Autodesk Inventor part; units mm, degrees
ref_plane "YZ Plane" through (0, 0, 0) normal (1, 0, 0) x (0, 1, 0)
ref_plane "XZ Plane" through (0, 0, 0) normal (0, 1, 0) x (-1, 0, 0)
ref_plane "XY Plane" through (0, 0, 0) normal (0, 0, 1) x (1, 0, 0)
sketch "Sketch4" plane through (0, 0, 0) normal (0, 1, 0) x (-1, 0, 0)
  line L0 (0, 0) -> (59.7662, 0)
  line L1 (59.7662, 0) -> (59.7662, -146.1262)
  line L2 (59.7662, -146.1262) -> (0, -146.1262)
  line L3 (0, -146.1262) -> (0, 0)
  line L4 (59.7662, 0) -> (53.4924, 0)
  line L5 (53.4924, 0) -> (53.4924, -9.5758)
  line L6 (53.4924, -9.5758) -> (59.7662, -9.5758)
  line L7 (59.7662, -9.5758) -> (59.7662, 0)
  line L8 (53.4924, -9.5758) -> (45.8724, -9.5758)
  line L9 (45.8724, -9.5758) -> (45.8724, -24.8158)
  line L10 (45.8724, -24.8158) -> (53.4924, -24.8158)
  line L11 (53.4924, -24.8158) -> (53.4924, -9.5758)
  line L12 (45.8724, -24.8158) -> (45.8724, -37.5158)
  line L13 (45.8724, -37.5158) -> (53.4924, -37.5158)
  line L14 (53.4924, -37.5158) -> (53.4924, -52.7558)
  line L15 (53.4924, -52.7558) -> (45.8724, -52.7558)
  line L16 (45.8724, -52.7558) -> (45.8724, -37.5158)
  line L17 (45.8724, -52.7558) -> (45.8724, -65.4558)
  line L18 (45.8724, -65.4558) -> (53.4924, -65.4558)
  line L19 (53.4924, -65.4558) -> (53.4924, -80.6958)
  line L20 (53.4924, -80.6958) -> (45.8724, -80.6958)
  line L21 (45.8724, -80.6958) -> (45.8724, -65.4558)
  line L22 (45.8724, -80.6958) -> (45.8724, -93.3958)
  line L23 (45.8724, -93.3958) -> (53.4924, -93.3958)
  line L24 (53.4924, -93.3958) -> (53.4924, -108.6358)
  line L25 (53.4924, -108.6358) -> (45.8724, -108.6358)
  line L26 (45.8724, -108.6358) -> (45.8724, -93.3958)
  line L27 (45.8724, -108.6358) -> (45.8724, -121.3358)
  line L28 (45.8724, -121.3358) -> (53.4924, -121.3358)
  line L29 (53.4924, -121.3358) -> (53.4924, -136.5758)
  line L30 (53.4924, -136.5758) -> (45.8724, -136.5758)
  line L31 (45.8724, -136.5758) -> (45.8724, -121.3358)
  line L32 (0, 0) -> (7.1628, 0)
  line L33 (7.1628, 0) -> (7.1628, -9.5758)
  line L34 (7.1628, -9.5758) -> (0, -9.5758)
  line L35 (0, -9.5758) -> (0, 0)
  line L36 (53.4924, -9.5758) -> (7.1628, -9.5758)
  line L37 (30.3276, -9.5758) -> (30.3276, -4.7879)
  line L38 (7.1628, -9.5758) -> (14.7828, -9.5758)
  line L39 (14.7828, -9.5758) -> (14.7828, -24.8158)
  line L40 (14.7828, -24.8158) -> (7.1628, -24.8158)
  line L41 (7.1628, -24.8158) -> (7.1628, -9.5758)
  line L42 (14.7828, -37.5158) -> (7.1628, -37.5158)
  line L43 (7.1628, -37.5158) -> (7.1628, -52.7558)
  line L44 (7.1628, -52.7558) -> (14.7828, -52.7558)
  line L45 (14.7828, -52.7558) -> (14.7828, -37.5158)
  line L46 (14.7828, -65.4558) -> (7.1628, -65.4558)
  line L47 (7.1628, -65.4558) -> (7.1628, -80.6958)
  line L48 (7.1628, -80.6958) -> (14.7828, -80.6958)
  line L49 (14.7828, -80.6958) -> (14.7828, -65.4558)
  line L50 (14.7828, -93.3958) -> (7.1628, -93.3958)
  line L51 (7.1628, -93.3958) -> (7.1628, -108.6358)
  line L52 (7.1628, -108.6358) -> (14.7828, -108.6358)
  line L53 (14.7828, -108.6358) -> (14.7828, -93.3958)
  line L54 (14.7828, -121.3358) -> (7.1628, -121.3358)
  line L55 (7.1628, -121.3358) -> (7.1628, -136.5758)
  line L56 (7.1628, -136.5758) -> (14.7828, -136.5758)
  line L57 (14.7828, -136.5758) -> (14.7828, -121.3358)
  line L58 (7.1628, -9.5758) -> (53.4924, -9.5758)
  line L59 (0, 0) -> (0, -146.1262)
  line L60 (0, -146.1262) -> (59.7662, -146.1262)
  line L61 (59.7662, -146.1262) -> (59.7662, 0)
  line L62 (62.9412, 0) -> (62.9412, -149.3012)
  line L63 (62.9412, -149.3012) -> (-3.175, -149.3012)
  line L64 (-3.175, -149.3012) -> (-3.175, 0)
  line L65 (0, 0.508) -> (59.7662, 0.508)
  line L66 (0, 3.683) -> (59.7662, 3.683)
  line L67 (62.9412, 0) -> (59.7662, 0)
  line L68 (59.7662, 0) -> (59.7662, 3.683)
  line L69 (59.7662, 3.683) -> (62.9412, 3.683)
  line L70 (62.9412, 3.683) -> (62.9412, 0)
  line L71 (-3.175, 0) -> (0, 0)
  line L72 (0, 0) -> (0, 3.683)
  line L73 (0, 3.683) -> (-3.175, 3.683)
  line L74 (-3.175, 3.683) -> (-3.175, 0)
  line L75 (0, 0.508) -> (0, 0.508)
  line L76 (0, 0.508) -> (0, 0)
  line L77 (0, 0) -> (0, 0)
  line L78 (0, 0) -> (0, 0.508)
  line L79 (59.7662, 0.508) -> (59.7662, 0.508)
  line L80 (59.7662, 0.508) -> (59.7662, 0)
  line L81 (59.7662, 0) -> (59.7662, 0)
  line L82 (59.7662, 0) -> (59.7662, 0.508)
  point P0 (59.7662, 0)
  dimension "d503" = 59.7662
  dimension "d504" = 146.1262
  dimension "d505" = 6.2738
  dimension "d506" = 9.5758
  dimension "d507" = 7.62
  dimension "d508" = 15.24
  dimension "d509" = 12.7
  dimension "d510" = 7.62
  dimension "d511" = 15.24
  dimension "d512" = 12.7
  dimension "d513" = 7.62
  dimension "d514" = 15.24
  dimension "d515" = 12.7
  dimension "d516" = 7.62
  dimension "d517" = 15.24
  dimension "d518" = 12.7
  dimension "d519" = 7.62
  dimension "d520" = 15.24
  dimension "d521" = 7.1628
  dimension "d522" = 9.5758
  dimension "d529" = 3.175
  dimension "d530" = 0.508
  dimension "d531" = 3.175
extrude "Extrusion4" add sketch "Sketch4" along normal blind 3.175 contours L72 L65 L68 L0 | L0 L33 L34 L3 | L3 L2 L1 L67 L62 L63 L64 L71 | L71 L74 L73 L72 | L0 L5 L8 L36 L33 | L34 L41 L40 L39 L36 L9 L10 L11 L6 L1 L2 L3 | L72 L66 L68 L65 | L0 L1 L6 L5 | L68 L69 L70 L67
sketch "Sketch5" plane through (0, 0, 0) normal (0, -1, 0) x (1, 0, 0)
  line L0 (-7.1628, -9.5758) -> (-14.7828, -9.5758)
  line L1 (-7.1628, -24.8158) -> (-7.1628, -9.5758)
  line L2 (-14.7828, -24.8158) -> (-7.1628, -24.8158)
  line L3 (-14.7828, -9.5758) -> (-14.7828, -24.8158)
  line L4 (-53.4924, -9.5758) -> (-53.4924, -24.8158)
  line L5 (-45.8724, -9.5758) -> (-53.4924, -9.5758)
  line L6 (-45.8724, -24.8158) -> (-45.8724, -9.5758)
  line L7 (-53.4924, -24.8158) -> (-45.8724, -24.8158)
  line L8 (-45.8724, -121.3358) -> (-53.4924, -121.3358)
  line L9 (-45.8724, -136.5758) -> (-45.8724, -121.3358)
  line L10 (-53.4924, -136.5758) -> (-45.8724, -136.5758)
  line L11 (-53.4924, -121.3358) -> (-53.4924, -136.5758)
  line L12 (-45.8724, -108.6358) -> (-45.8724, -93.3958)
  line L13 (-53.4924, -108.6358) -> (-45.8724, -108.6358)
  line L14 (-53.4924, -93.3958) -> (-53.4924, -108.6358)
  line L15 (-45.8724, -93.3958) -> (-53.4924, -93.3958)
  line L16 (-45.8724, -80.6958) -> (-45.8724, -65.4558)
  line L17 (-53.4924, -80.6958) -> (-45.8724, -80.6958)
  line L18 (-53.4924, -65.4558) -> (-53.4924, -80.6958)
  line L19 (-45.8724, -65.4558) -> (-53.4924, -65.4558)
  line L20 (-45.8724, -52.7558) -> (-45.8724, -37.5158)
  line L21 (-53.4924, -52.7558) -> (-45.8724, -52.7558)
  line L22 (-53.4924, -37.5158) -> (-53.4924, -52.7558)
  line L23 (-45.8724, -37.5158) -> (-53.4924, -37.5158)
  line L24 (-7.1628, -80.6958) -> (-7.1628, -65.4558)
  line L25 (-14.7828, -80.6958) -> (-7.1628, -80.6958)
  line L26 (-14.7828, -65.4558) -> (-14.7828, -80.6958)
  line L27 (-7.1628, -65.4558) -> (-14.7828, -65.4558)
  line L28 (-14.7828, -121.3358) -> (-14.7828, -136.5758)
  line L29 (-7.1628, -121.3358) -> (-14.7828, -121.3358)
  line L30 (-7.1628, -136.5758) -> (-7.1628, -121.3358)
  line L31 (-14.7828, -136.5758) -> (-7.1628, -136.5758)
  line L32 (-14.7828, -37.5158) -> (-14.7828, -52.7558)
  line L33 (-7.1628, -37.5158) -> (-14.7828, -37.5158)
  line L34 (-7.1628, -52.7558) -> (-7.1628, -37.5158)
  line L35 (-14.7828, -52.7558) -> (-7.1628, -52.7558)
  line L36 (-7.1628, -108.6358) -> (-7.1628, -93.3958)
  line L37 (-14.7828, -108.6358) -> (-7.1628, -108.6358)
  line L38 (-14.7828, -93.3958) -> (-14.7828, -108.6358)
  line L39 (-7.1628, -93.3958) -> (-14.7828, -93.3958)
  line L40 (-3.048, -3.048) -> (-3.048, -143.0782)
  line L41 (-3.048, -143.0782) -> (-56.7182, -143.0782)
  line L42 (-56.7182, -143.0782) -> (-56.7182, -3.048)
  line L43 (-56.7182, -3.048) -> (-3.048, -3.048)
  line L44 (-62.9412, 3.683) -> (3.175, 3.683)
  line L45 (3.175, 3.683) -> (3.175, -149.3012)
  line L46 (3.175, -149.3012) -> (-62.9412, -149.3012)
  line L47 (-62.9412, -149.3012) -> (-62.9412, 3.683)
  line L48 (0, 0.508) -> (-59.7662, 0.508)
  line L49 (-59.7662, 0.508) -> (-59.7662, -146.1262)
  line L50 (-59.7662, -146.1262) -> (0, -146.1262)
  line L51 (0, -146.1262) -> (0, 0.508)
  point P0 (0, 0)
  dimension "d532" = 3.175
extrude "Extrusion5" add sketch "Sketch5" along normal blind 8.89 contours L44 L45 L46 L47
properties part number "RelayCaseTop" material "Rubber, Silicone"
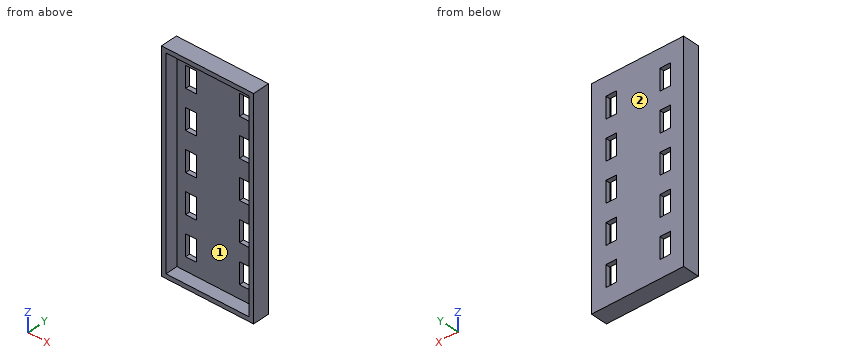
Could you check a few things on this model? Use its own coordinates, in mm. Face numbers are marked on the shaded views. Give positions to 0.01 mm unless a question says otherwise; leave off trailing zeros. Order: outer loops, then holes, each group sorted by start corner. A loop starts at its lowest first (then second) coordinate and runs counter-clockwise, first axis right, second up. Notation, with made-up numbers: M -4,-20 L 54,-20 A25 ccw 54,9 Z; hole C 2.5,74 d8. An arc over 180 degrees is marked long. One line per question, with ' | ' between items.
1. I want a section at D-D (z = -138). List the corners of the cut face in (x, y) for me (3 decimals), and give its area (3 significant figures).
Results:
outline: M -62.941,-8.89 L -59.766,-8.89 L -59.766,0 L 0,0 L 0,-8.89 L 3.175,-8.89 L 3.175,3.175 L -62.941,3.175 Z | area: 266 mm²
2. I want a section at B-B (x = -48.5). List the corners of the cut face in (y, z) for me (3 decimals), and give its area (3 significant figures).
Results:
outline: M -8.89,-149.301 L 3.175,-149.301 L 3.175,-136.576 L 0,-136.576 L 0,-146.126 L -8.89,-146.126 Z; M -8.89,0.508 L 0,0.508 L 0,-9.576 L 3.175,-9.576 L 3.175,3.683 L -8.89,3.683 Z; M 0,-121.336 L 3.175,-121.336 L 3.175,-108.636 L 0,-108.636 Z; M 0,-93.396 L 3.175,-93.396 L 3.175,-80.696 L 0,-80.696 Z; M 0,-65.456 L 3.175,-65.456 L 3.175,-52.756 L 0,-52.756 Z; M 0,-37.516 L 3.175,-37.516 L 3.175,-24.816 L 0,-24.816 Z | area: 300 mm²
3. I want a section at C-C (y = -3.5). List the corners of the cut face in (x, z) for me (3 decimals).
Results:
outline: M -62.941,-149.301 L 3.175,-149.301 L 3.175,3.683 L -62.941,3.683 Z; hole M -59.766,-146.126 L 0,-146.126 L 0,0.508 L -59.766,0.508 Z
4. I'm going to push a flat-ended pin straight in: pin 1 (8 mm diameter, centred on x = -30.5, z = -13.5, fed in from -Y). Where does the tip first touch, or does it pass through?
Results:
pin 1: y = 0
5. I want a section at A-A (z = -71). List the corners of the cut face in (x, y) for me (3 decimals).
Results:
outline: M -62.941,-8.89 L -59.766,-8.89 L -59.766,0 L -53.492,0 L -53.492,3.175 L -62.941,3.175 Z; M -45.872,0 L -14.783,0 L -14.783,3.175 L -45.872,3.175 Z; M -7.163,0 L 0,0 L 0,-8.89 L 3.175,-8.89 L 3.175,3.175 L -7.163,3.175 Z
6. We'd pull the mould along X, two halves only. Please class the marked faces 1 and 2: +X half, -X half, draft (parallel to the pull), parting line (faces both ways), or undercut.
Results:
face 1: undercut | face 2: draft
7. If I drill on line 1 (X direction, y = 1, z = -99) (3 decimals); line 2 (Z direction, x = -12.5, y = 1.25); line 3 (Z direction, x = -11, y = -0.5), over which ranges is the centre line in solid material (lowest first)?
Results:
line 1: -62.941 to -53.492, -45.872 to -14.783, -7.163 to 3.175 | line 2: -149.3 to -136.58, -121.34 to -108.64, -93.4 to -80.7, -65.46 to -52.76, -37.52 to -24.82, -9.58 to 3.68 | line 3: -149.3 to -146.13, 0.51 to 3.68
